Input: part model. Units: mm. Frame: model coordinates. Face numbers are marked on the shaded views. A direction names the side the tool comes from. Give positions to 0.01 mm unless a question says otherwise; leave off trailing zeros. Order: outer loops, then holes, each group sorted by start corner. A loop starts at its lowest first (then second) coordinate and runs counter-clockwise, first axis right, second up. Notation, with made-up numbers: (21.25, 84.25) -> (78.25, 84.25) arc R34 ccw to (78.25, 122.25) -> close; hole circle Ø4 at (55, 77.25). An arc over 180 degrees is marked (long way). Use a Markdown table: item, result. Add a question column.
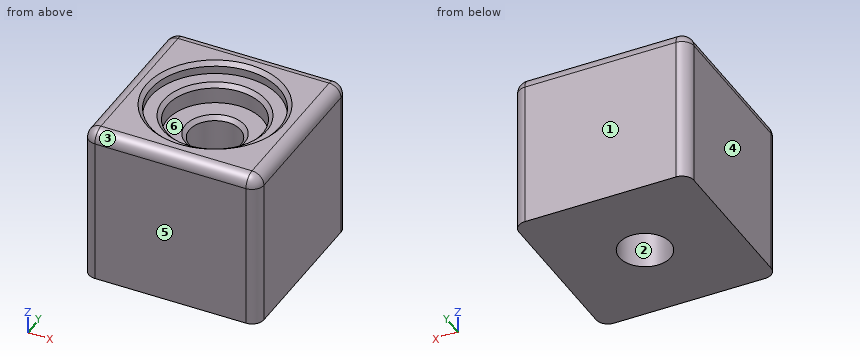
Autodesk Fusion 360 part; units mm, degrees
sketch "Sketch1" plane through (0, 0, 0) normal (0, 0, 1) x (1, 0, 0)
  line L0 (0, 0) -> (-44, 0)
  line L1 (-44, 0) -> (-44, 44)
  line L2 (-44, 44) -> (0, 44)
  line L3 (0, 44) -> (0, 0)
  dimension "d1" = 44
  dimension "d2" = 44
extrude "Extrude1" add sketch "Sketch1" along normal blind 40
sketch "Sketch2" plane through (0, 0, 40) normal (0, 0, 1) x (-1, 0, 0)
  line L0 (0, -44) -> (44, -44)
  line L1 (44, -44) -> (44, 0)
  line L2 (44, 0) -> (0, 0)
  line L3 (0, 0) -> (0, -44)
  line L4 (44, -44) -> (0, 0)
  line L5 (0, -44) -> (44, 0)
  circle A0 centre (22, -22) radius 16.25
  dimension "d5" = 32.5
extrude "Extrude2" cut sketch "Sketch2" against normal blind 3 contours L4 L5 A0 | L4 L5 A0 | L4 L5 A0 | L4 L5 A0
sketch "Sketch3" plane through (0, 0, 37) normal (0, 0, 1) x (-1, 0, 0)
  circle A0 centre (22, -22) radius 16.25
  circle A1 centre (22, -22) radius 12
  dimension "d8" = 24
extrude "Extrude3" cut sketch "Sketch3" against normal blind 5 contours A1
sketch "Sketch4" plane through (0, 0, 32) normal (0, 0, 1) x (-1, 0, 0)
  circle A0 centre (22, -22) radius 12
  circle A1 centre (22, -22) radius 6.45
  dimension "d11" = 12.9
extrude "Extrude4" cut sketch "Sketch4" against normal blind 50 contours A1
fillet "Fillet1" radius 3 8 edges at (-22, 44, 40) (-44, 22, 40) (-22, 0, 40) (0, 22, 40) (0, 0, 20) (-44, 0, 20) (0, 44, 20) (-44, 44, 20)
chamfer "Chamfer1" distance 1 angle 45 3 edges at (-10.8121, 17.6606, 37) (-15.9865, 19.6676, 32) (-6.8497, 16.1237, 40)
Q1. First-contact query: pin 1 (19 mm diameter, centred on x = -18.5, y = 18.5, fed in from +Z); pin 2 (1.5 mm diameter, centred on x = -10.5, y = 19, fed in from +Z); pin 3 (15 mm diameter, centred on x = -22, y = 22, fed in from +Z). Flat tips, straight axial feed; report the tip coordinate or a pass-through.
Q2. Draft query along Y for the marked faces 1, 2, 3 and 4. Return one class per face: +Y half, -Y half, draft (parallel to the pull), parting line (faces both ways), or undercut.
Q3. Section query B-B (y = 22). Return loops of the section in (x, z).
Q4. Ray query, line 1 (Y direction, x = -22, z = 33.05); line 2 (X direction, y = 22, z = 20); line 3 (X direction, y = 22, z = 34). Return the intervals inside material, ascending.
Q5. Section query C-C (z = 24). Return loops of the section in (x, y), plus the area to 3 significant figures.
Q6. Access query for the marked faces 5 and 6. Directions: +Z, -Z, +X, -X, +Y, -Y. A direction counts if a zero-diameter tool reaches every point of the face in a straight line with its end or side. Return the directions, or none.
Q7. Section query A-A (x = -22). Return loops of the section in (y, z), plus the area to 3 significant figures.
Solution:
| question | item | result |
|---|---|---|
| 1 | pin 1 | stops at z = 37 |
| 1 | pin 2 | stops at z = 36.63 |
| 1 | pin 3 | stops at z = 32 |
| 2 | face 1 | +Y half |
| 2 | face 2 | undercut |
| 2 | face 3 | -Y half |
| 2 | face 4 | draft |
| 3 | outline | (-44, 0) -> (-28.45, 0) -> (-28.45, 31) -> (-29.45, 32) -> (-34, 32) -> (-34, 36) -> (-35, 37) -> (-38.25, 37) -> (-38.25, 39) -> (-39.25, 40) -> (-41, 40) arc R3 ccw to (-44, 37) -> close; (-15.55, 0) -> (0, 0) -> (0, 37) arc R3 ccw to (-3, 40) -> (-4.75, 40) -> (-5.75, 39) -> (-5.75, 37) -> (-9, 37) -> (-10, 36) -> (-10, 32) -> (-14.55, 32) -> (-15.55, 31) -> close |
| 4 | line 1 | y = 0 to 10, 34 to 44 |
| 4 | line 2 | x = -44 to -28.45, -15.55 to 0 |
| 4 | line 3 | x = -44 to -34, -10 to 0 |
| 5 | outline | (-44, 3) arc R3 ccw to (-41, 0) -> (-3, 0) arc R3 ccw to (0, 3) -> (0, 41) arc R3 ccw to (-3, 44) -> (-41, 44) arc R3 ccw to (-44, 41) -> close; hole circle Ø12.9 at (-22, 22) |
| 5 | area | 1,800 mm² |
| 6 | face 5 | +Z, -Z, +X, -X, -Y |
| 6 | face 6 | +Z |
| 7 | outline | (0, 0) -> (15.55, 0) -> (15.55, 31) -> (14.55, 32) -> (10, 32) -> (10, 36) -> (9, 37) -> (5.75, 37) -> (5.75, 39) -> (4.75, 40) -> (3, 40) arc R3 ccw to (0, 37) -> close; (28.45, 0) -> (44, 0) -> (44, 37) arc R3 ccw to (41, 40) -> (39.25, 40) -> (38.25, 39) -> (38.25, 37) -> (35, 37) -> (34, 36) -> (34, 32) -> (29.45, 32) -> (28.45, 31) -> close |
| 7 | area | 1,120 mm² |
